```python
from build123d import *

# Parameters (mm, degrees)
ESQUISSE1_R        = 1.5
BOSS_EXTRU_1_DEPTH = 3


with BuildPart() as part:
    # Esquisse1 → Boss.-Extru.1 (new body)
    with BuildSketch(Plane.XZ.offset(3)):
        Polygon((2.350913118, -2.544249892), (3.378841599, 0.763825536), (1.027928481, 3.308075428), (-2.350913118, 2.544249892), (-3.378841599, -0.763825536), (-1.027928481, -3.308075428), align=None)
        with Locations(Location((0, 0, 0), (0, 0, 90))):
            Circle(ESQUISSE1_R, mode=Mode.SUBTRACT)
    extrude(amount=-BOSS_EXTRU_1_DEPTH)


solid = part.part
```
For this review, take the finished solid that the model builds, in its own axes (mm). Coordinates: 2 decimals unless noted, no trailing zeros. Order: outer loops, then holes, each group sorted by start corner. A loop starts at its lowest first (then second) coordinate and runs counter-clockwise, first axis right, second up. Notation, with made-up numbers: (-28, 27) - (-13, 27) arc R19 ccw to (-13, 56) - close; hole circle Ø1 at (-28.5, 68). An arc over 180 degrees is marked (long way). Answer as a JSON object with one key per item and string values. Group by question number.
1. We need section A-A on z = 0. State the section outline as (x, y) points, then the cut area to 3 significant figures.
2. We need section B-B on x = 0. State the section outline as (y, z) points.
3. We need section C-C on y = -2.65. State the section outline as (x, z) points.
4. For probe 1 along X at (y, z) = (-1.2, 0); probe 2 along Z at (x, y) = (-0.75, -0.95); probe 3 along X at (y, z) = (-2.45, 1), list the stretches that pass through material, from the lowest coordinate up.
5. We need section D-D on z = 2. State the section outline as (x, y) points.
Final values:
{
 "1": {"outline": "(-3.14, -3) - (-1.5, -3) - (-1.5, 0) - (-3.14, 0) - close; (1.5, -3) - (3.14, -3) - (3.14, 0) - (1.5, 0) - close", "area": "9.85 mm²"},
 "2": {"outline": "(-3, -3.08) - (0, -3.08) - (0, -1.5) - (-3, -1.5) - close; (-3, 1.5) - (0, 1.5) - (0, 3.08) - (-3, 3.08) - close"},
 "3": {"outline": "(-3.38, -0.76) - (-1.03, -3.31) - (2.35, -2.54) - (3.38, 0.76) - (1.03, 3.31) - (-2.35, 2.54) - close; hole circle Ø3 at (0, 0)"},
 "4": {"probe 1": "-3.14 to -1.5, 1.5 to 3.14", "probe 2": "-3.25 to -1.3, 1.3 to 2.91", "probe 3": "-2.83 to -1.12, 1.12 to 3.16"},
 "5": {"outline": "(-2.52, -3) - (2.24, -3) - (2.24, 0) - (-2.52, 0) - close"}
}
